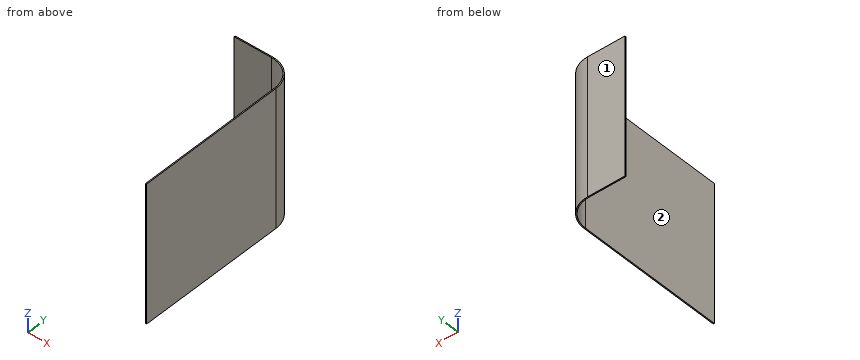
Autodesk Inventor part; units mm, degrees
ref_plane "YZ Plane" through (0, 0, 0) normal (1, 0, 0) x (0, 1, 0)
ref_plane "XZ Plane" through (0, 0, 0) normal (0, 1, 0) x (-1, 0, 0)
ref_plane "XY Plane" through (0, 0, 0) normal (0, 0, 1) x (1, 0, 0)
sketch "Sketch1" plane through (0, 0, 0) normal (0, 0, 1) x (1, 0, 0)
  line L0 (-140, 100) -> (0, 100)
  arc A0 (100, 0) -> (0, 100) centre (0, 0) ccw
  line L1 (100, 0) -> (100, -560)
  line L2 (100, -560) -> (96, -560)
  line L3 (96, -560) -> (96, 0)
  arc A1 (96, 0) -> (0, 96) centre (0, 0) ccw
  line L4 (0, 96) -> (-140, 96)
  line L5 (-140, 96) -> (-140, 100)
  dimension "d0" = 4
  dimension "d1" = 660
  dimension "d2" = 240
  dimension "d3" = 100
extrude "Extrusion1" add sketch "Sketch1" along normal mid plane 520
properties part number "RT_FRM_MC_012_Electrical_housing_door" material "Polycarbonate, Clear"
Part model, mm, in its own coordinate system. Face numbers are marked on the shaded views. A direction names the side the tool comes from. Coordinates: 2 decimals unless noted, no trailing zeros. Order: outer loops, then holes, each group sorted by start corner. A loop starts at its lowest first (then second) coordinate and runs counter-clockwise, first axis right, second up.
(1) Pin check, flat tips, straight feed: pin 1 Ø10 at (x, z) = (73, 199.5) entering from -Y; pin 2 Ø6 at (x, z) = (-22, 202.5) entering from -Y. Stop position of each tip, or through.
Check sheet entries:
pin 1: stops at y = 55.96
pin 2: stops at y = 96
(2) Slice it at B-B, the plane y = -357. Write the cut outline in (x, z), and give its area (3 significant figures).
Check sheet entries:
outline: (96, -260) - (100, -260) - (100, 260) - (96, 260) - close
area: 2,080 mm2
(3) Probe L1, parallel to Y at x = -101, z = -151; L2, parallel to X at y = 30.5, z = -17.5. List the from-to ranges inside material, lowest first.
Check sheet entries:
L1: y = 96 to 100
L2: x = 91.03 to 95.24
(4) Slice it at A-A, the plane z = 41. Write the cut outline in (x, y).
Check sheet entries:
outline: (-140, 96) - (0, 96) arc R96 cw to (96, 0) - (96, -560) - (100, -560) - (100, 0) arc R100 ccw to (0, 100) - (-140, 100) - close
(5) Tool access for the marked faces 1 and 2: list every direction of +Z, -Z, +X, -X, +Y, -Y with a clear straight run to the whole face (end or side of a thin tool).
Check sheet entries:
face 1: +Z, -Z, +X, -X, +Y
face 2: +Z, -Z, -X, -Y
